```python
from build123d import *

# Parameters (mm, degrees)
SKETCH1_R           = 4.7625
BOSS_EXTRUDE1_DEPTH = 3.175
SKETCH2_R           = 6.35
BOSS_EXTRUDE2_DEPTH = 105.4492
SKETCH3_R           = 4.7625
BOSS_EXTRUDE3_DEPTH = 3.175
SKETCH5_R           = 1.518393352
CUT_EXTRUDE1_DEPTH  = 194.727414479


with BuildPart() as part:
    # Sketch1 → Boss-Extrude1 (new body)
    with BuildSketch(Plane.XY):
        with BuildLine():
            Line((0, 0), (150, 0))
            ThreePointArc((150, 0), (157.5, 7.5), (150, 15))
            Line((150, 15), (-15, 15))
            ThreePointArc((-15, 15), (-10.606601718, 4.393398282), (0, 0))
        make_face()
        with Locations((15, 7.5)):
            Circle(SKETCH1_R, mode=Mode.SUBTRACT)
    extrude(amount=BOSS_EXTRUDE1_DEPTH)

    # Sketch2 → Boss-Extrude2 (add)
    with BuildSketch(Plane.XY.offset(3.175)):
        with Locations(Location((150, 7.5, 0), (0, 0, 180))):
            Circle(SKETCH2_R)
    extrude(amount=BOSS_EXTRUDE2_DEPTH)

    # Sketch3 → Boss-Extrude3 (add)
    with BuildSketch(Plane.XY.offset(108.6242)):
        with BuildLine():
            Line((0, 0), (150, 0))
            ThreePointArc((150, 0), (157.5, 7.5), (150, 15))
            Line((150, 15), (-15, 15))
            ThreePointArc((-15, 15), (-10.606601718, 4.393398282), (0, 0))
        make_face()
        with Locations((15, 7.5)):
            Circle(SKETCH3_R, mode=Mode.SUBTRACT)
    extrude(amount=BOSS_EXTRUDE3_DEPTH)

    # Sketch5 → Cut-Extrude1 (cut, through all)
    with BuildSketch(Plane.XY.offset(111.7992)):
        with Locations((150, 7.5)):
            Circle(SKETCH5_R)
        with BuildLine():
            Line((57.017518256, 0), (77.982481744, 0))
            ThreePointArc((77.982481744, 0), (76.202985115, 1.025330402), (75.5, 2.955025356))
            ThreePointArc((75.5, 2.955025356), (67.5, 10.955025356), (59.5, 2.955025356))
            ThreePointArc((59.5, 2.955025356), (58.797014885, 1.025330402), (57.017518256, 0))
        make_face()
    extrude(amount=-CUT_EXTRUDE1_DEPTH, mode=Mode.SUBTRACT)


solid = part.part
```
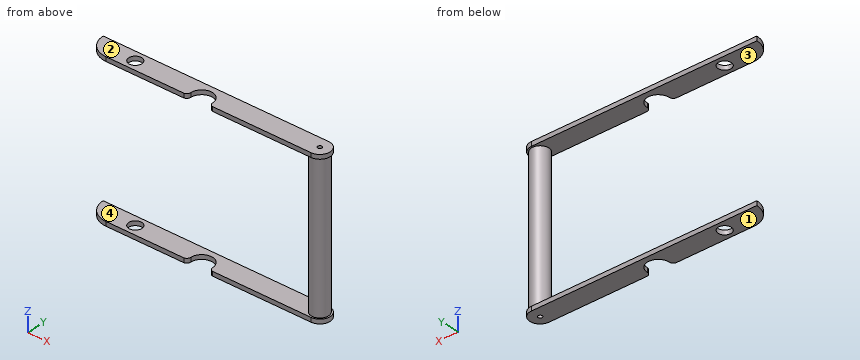
Build history of the part. All positions in model axes, mm. Face numbers are marked on the shaded views. Give positions to 0.01 mm unless a question says otherwise; leave off trailing zeros. Order: outer loops, then holes, each group sorted by start corner. A loop starts at its lowest first (then second) coordinate and runs counter-clockwise, first axis right, second up. Notation, with made-up numbers: M 78,-27.75 L 117,-27.75 A23 cw 117,5.25 Z; hole C 55.25,-30 d11. An arc over 180 degrees is marked long. Return JSON: item names as keys, results as strings.
Q1. Wall check: probe 1 along Z at (x, y) = (30.5, 7) (3 decimals); probe 2 along Y at (x, z) = (15, 109); probe 3 along X at (y, z) = (3, 59). Give the ranges that are in metal, low to high. Write a range as from..to.
Answer list:
{"probe 1": "z = 0..3.175, 108.624..111.799", "probe 2": "y = 0..2.74, 12.26..15", "probe 3": "x = 145.52..154.48"}
Q2. Band-saw the part on C-C (z = 105). Give the cut face in (x, y).
Answer list:
{"outline": "C 150,7.5 d12.7; hole C 150,7.5 d3.04"}
Q3. Band-saw the part on A-A (x = 91). Give the cut face in (y, z) (3 decimals).
Answer list:
{"outline": "M 0,0 L 15,0 L 15,3.175 L 0,3.175 Z; M 0,108.624 L 15,108.624 L 15,111.799 L 0,111.799 Z"}
Q4. Two-plate mould, pull along Z, no slides. Class the marked faces 1, 2, 3 and 4: pulls with the +Z half, pulls with the -Z half, needs draft (parallel to the pull), parting line crosses it, or undercut.
Answer list:
{"face 1": "pulls with the -Z half", "face 2": "pulls with the +Z half", "face 3": "undercut", "face 4": "undercut"}
Q5. Flat gauge pin, fed straight in: pin 1 (5 mm diameter, centred on y = 11, z = 50, fed in from -X). Where does the tip first touch, or does it go through?
Answer list:
{"pin 1": "stops at x = 143.73"}
Q6. Band-saw the part on B-B (x = 15). Give the cut face in (y, z) (1 decimal).
Answer list:
{"outline": "M 0,0 L 2.7,0 L 2.7,3.2 L 0,3.2 Z; M 0,108.6 L 2.7,108.6 L 2.7,111.8 L 0,111.8 Z; M 12.3,0 L 15,0 L 15,3.2 L 12.3,3.2 Z; M 12.3,108.6 L 15,108.6 L 15,111.8 L 12.3,111.8 Z"}
